Here's how the part is built. I have some questions about the finished solid (model axes, mm). A direction names the side the tool comes from. Coordinates: 2 decimals unless noted, no trailing zeros. Order: outer loops, then holes, each group sorted by start corner. A loop starts at its lowest first (then second) coordinate and runs counter-clockwise, first axis right, second up. Notation, with made-up numbers: M 55,60.5 L 114,60.5 A29 ccw 114,85.5 Z; hole C 79.25,2.25 d1. An arc over 180 degrees is marked long. One line per question, with ' | ' between items. Start each with the question number.
```python
from build123d import *

# Parameters (mm, degrees)
F0_R     = 2.15
F1_DEPTH = 11.4
F3_DEPTH = 10
F4_R     = 6
F6_DEPTH = 25
F7_R     = 1


with BuildPart() as f1:
    # F0 (on Front) → F1 (new body, symmetric)
    with BuildSketch(Plane.XZ):
        with BuildLine():
            Line((-22, -6), (0, -6))
            ThreePointArc((0, -6), (6, 0), (0, 6))
            Line((0, 6), (-12, 6))
            Line((-12, 6), (-12, 2))
            Line((-12, 2), (-22, 2))
            Line((-22, 2), (-22, -6))
        make_face()
        Circle(F0_R, mode=Mode.SUBTRACT)
    extrude(amount=F1_DEPTH, both=True)

    # F2 (on Front) → F3 (cut, symmetric)
    with BuildSketch(Plane.XZ):
        with BuildLine():
            Line((-26.315558, 9.79657), (-26.315558, -3.972946))
            ThreePointArc((-26.315558, -3.972946), (-10.728351, -0.64123), (1.317963, 9.79657))
            Line((1.317963, 9.79657), (-26.315558, 9.79657))
        make_face()
    extrude(amount=F3_DEPTH, both=True, mode=Mode.SUBTRACT)

    # F4
    f4_edges = [f1.edges().sort_by_distance(p)[0] for p in [
        (-10.985467, 10, -0.767914),
        (-10.985467, -10, -0.767914),
    ]]
    fillet(f4_edges, radius=F4_R)

    # F5 (on face) → F6 (cut)
    with BuildSketch(Plane(origin=(0, 0, -6), x_dir=(1, 0, 0), z_dir=(0, 0, -1))):
        with BuildLine():
            Line((-13, 3), (-16.800034, 3))
            ThreePointArc((-16.800034, 3), (-18.707277, 7.186787), (-22, 10.4))
            Line((-22, 10.4), (-22, -10.4))
            ThreePointArc((-22, -10.4), (-18.707277, -7.186787), (-16.800034, -3))
            Line((-16.800034, -3), (-13, -3))
            Line((-13, -3), (-13, 3))
        make_face()
    extrude(amount=-F6_DEPTH, mode=Mode.SUBTRACT)

    # F7
    f7_edges = [f1.edges().sort_by_distance(p)[0] for p in [
        (-6, -11.4, 6),
        (-11, 11.4, -6),
    ]]
    fillet(f7_edges, radius=F7_R)


solid = f1.part
```
1. Which directions (+Z, -Z, +X, -X, +Y, -Y) give clear straight access to the entire face, cutting with the end or side of a thin tool? Please do faces 4 (the face through (-17, -11, 2)), 5 (the face through (-19.37, 8.05, -3.83)), 6 (the face through (-7.2, -0.056, 1.407)).
2. Will these pins go through, and if not, where does the flat tip stop? pin 1 (0.6 mm diameter, centred on x = -11.5, z = 5.5, fed in from +Y); pin 2 (1.8 mm diameter, centred on y = 10.5, z = 4.5, fed in from -X); pin 3 (0.7 mm diameter, centred on x = -17.5, y = -10, fed in from +Z).
3. Imagine slicing it at A-A (y = -1.25). List the corners of the cut face in (x, z) for me.
4. I need wall thicknesses on line 1 (Z direction, x = 0, y = 1); line 2 (Y direction, x = -9.25, z = 2.5); line 3 (Y direction, x = -20, z = -2.75). Which ranges of each line are inside material? Lowest first, please.
5. Imagine slicing it at B-B (y = -7.25). List the corners of the cut face in (x, z) for me.
6. We'd pull the mould along Y, two halves only. Please class faces 1 (the face through (-10.846, -11.115, -5.699)), 2 (the face through (-15, -3, -4)), 3 (the face through (6, 0, 0)): released by +Y, released by -Y, zero draft, split by the parting line, or undercut.
Entries:
1) face 4: +Z, -X, +Y, -Y | face 5: +Z, -Z, -X | face 6: +Z, -X
2) pin 1: y = 11.38 | pin 2: x = -12 | pin 3: z = 2
3) outline: M -13,-6 L 0,-6 A6 ccw 0,6 L -1.76,6 A32 cw -13,-1.66 Z; hole C 0,0 d4.3
4) line 1: -6 to -2.15, 2.15 to 6 | line 2: -11.4 to -8.5, 8.5 to 11.4 | line 3: -11.4 to -8.74, 8.74 to 11.4
5) outline: M -18.75,-6 L 0,-6 A6 ccw 0,6 L -3.1,6 A31.04 cw -18.75,-2.41 Z; hole C 0,0 d4.3
6) face 1: released by -Y | face 2: undercut | face 3: zero draft
